Design review of the part shown in the three views and the two pictorial views. Dimensions are in mm from the part's minimum x, y and z. Round coordinates to 2 decimals unless told otherwise and drop trailing zeros. Loops run counter-clockwise (first coordinate to the right, second up) from the corner with the lowest first, then second, coordinate; pieces in that order, holes last. Notation, with made-up numbers: M 3,-33.75 L 45,-33.75 A16 cw 45,-18.75 Z; hole C 38,16.25 d5. An arc over 180 degrees is marked long. One line per question, with ' | ' between items. Start each with the question number.
1) We need section A-A (y = 4). Give the boundary of the cut face in (x, z), and give its area (3 significant figures).
2) We need section D-D (x = 2). Give the boundary of the cut face in (y, z), and give its area (3 significant figures).
3) For probe 1 along Y at (x, z) = (4, 2); probe 2 along X at (y, z) = (4.75, 8.25), list the stretches that pass through material, from the lowest coordinate up. Write a range as from..to.
4) We need section C-C (z = 4.5). Give the boundary of the cut face in (x, y), and give its area (3 significant figures).
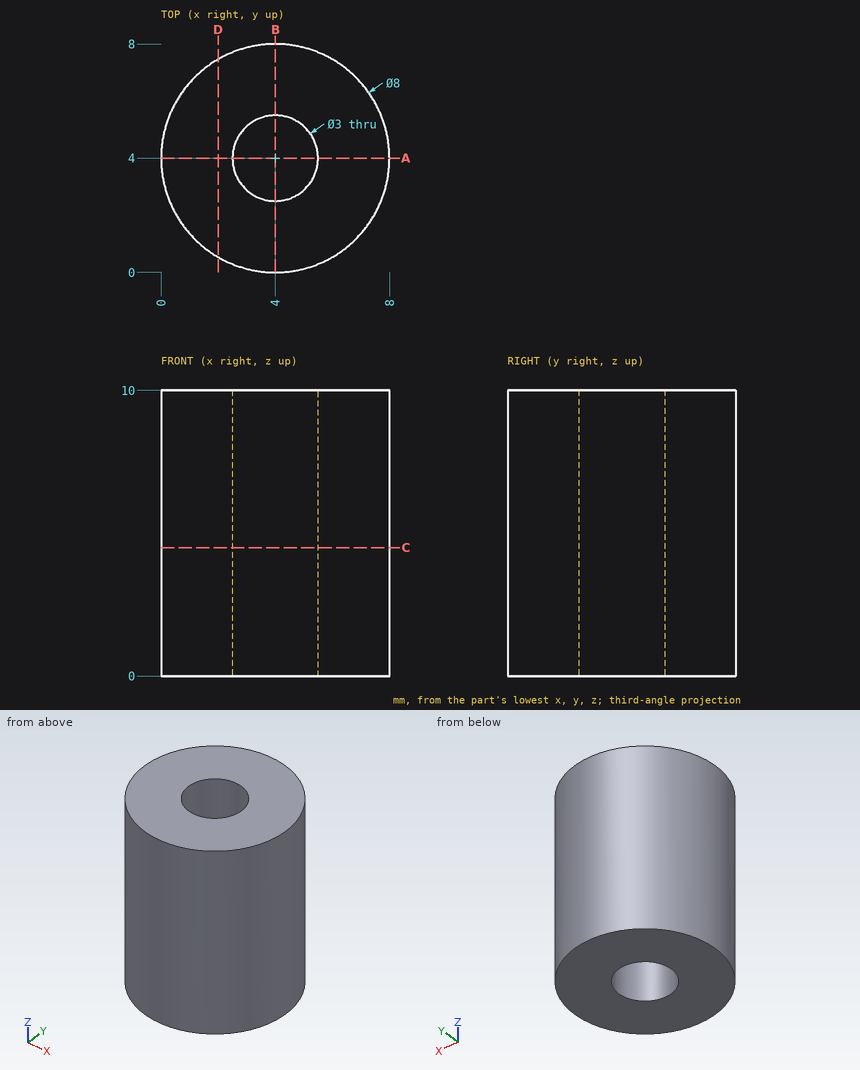
Answers below:
1) outline: M 0,0 L 2.5,0 L 2.5,10 L 0,10 Z; M 5.5,0 L 8,0 L 8,10 L 5.5,10 Z | area: 50.0 mm^2
2) outline: M 0.54,0 L 7.46,0 L 7.46,10 L 0.54,10 Z | area: 69.3 mm^2
3) probe 1: 0..2.5, 5.5..8 | probe 2: 0.07..2.7, 5.3..7.93
4) outline: C 4,4 d8; hole C 4,4 d3 | area: 43.2 mm^2
